Work out the finished part from the listing and answer in its coordinate system (mm). A direction names the side the tool comes from. Round coordinates to 2 decimals unless told otherwise and drop trailing zeros. Write each loop counter-clockwise with the first axis right and the second up, starting at its lowest first coordinate (ties: lowest second). Pieces come first, ordered by that corner, then holes. Notation, with made-up numbers: M 83,-5.75 L 105,-5.75 A23 ccw 105,10.25 Z; hole C 29,7 d9. An arc over 180 degrees is marked long. One line per item, written item: value. Start each with the question number.
Q1. Consider probe 1 along Y at (x, z) = (-234.5, -166); probe 2 along Y at (x, z) = (-195, -372). Determine where each line is inside the solid, lowest interval first.
Q2. Find section C-C (z = -253). Write down the section's boundary in (x, y), and give its area (3 significant figures).
Q3. Given pin 1 Ø6 at (x, y) = (-205.5, 136) entering from -Z; pin 2 Ø16 at (x, z) = (-109.5, -424) entering from -Y; pin 3 Ø4 at (y, z) = (30, -283) entering from +X; pin 4 Ø6 at (x, z) = (-209, -417) entering from +Y, each flat-ended and moving along its own axis, determine where each tip first touches the part or whether it passes through.
Q4. Find section A-A (x = -243.5). Write down the section's boundary in (y, z), and give its area (3 significant figures).
Q5. A tool of negligible diameter and unlimited length cuts with its end or side. For faces 1 (the flat face through (-173, 140, -412)), 2 (the flat face through (-173, 57, -412)), 3 (the flat face through (-350, 59, -309)), from which of +Z, -Z, +X, -X, +Y, -Y can it reach the whole face along a straight path? Write none if from no direction.
Q6. Find section B-B (y = 33.5). Write down the section's boundary in (x, z).
from build123d import *

# Parameters (mm, degrees)
BOSS_EXTRUDE1_DEPTH = 350
SKETCH3_W           = 350
SKETCH3_H           = 15
BOSS_EXTRUDE2_DEPTH = 20


with BuildPart() as part:
    # Sketch1 → Boss-Extrude1 (new body)
    with BuildSketch(Plane(origin=(0, 0, 0), x_dir=(0, 0, -1), z_dir=(1, 0, 0))):
        Polygon((0, 0), (412, 0), (412, 149.955736518), align=None)
    extrude(amount=-BOSS_EXTRUDE1_DEPTH)

    # Sketch3 → Boss-Extrude2 (add)
    with BuildSketch(Plane(origin=(0, 0, -412), x_dir=(-1, 0, 0), z_dir=(0, 0, -1))):
        with Locations((175, 122.455736518)):
            Rectangle(SKETCH3_W, SKETCH3_H)
    extrude(amount=BOSS_EXTRUDE2_DEPTH)


solid = part.part
The answers:
1. probe 1: 0 to 60.42
1. probe 2: 0 to 135.4
2. outline: M -350,0 L 0,0 L 0,92.08 L -350,92.08 Z
2. area: 32,200 mm2
3. pin 1: z = -412
3. pin 2: y = 114.96
3. pin 3: x = 0
3. pin 4: y = 129.96
4. outline: M 0,-412 L 114.96,-412 L 114.96,-432 L 129.96,-432 L 129.96,-412 L 149.96,-412 L 0,0 Z
4. area: 31,200 mm2
5. face 1: -Z, +X, -X, +Y
5. face 2: -Z, +X, -X, -Y
5. face 3: +Z, -Z, -X, +Y, -Y
6. outline: M -350,-412 L 0,-412 L 0,-92.04 L -350,-92.04 Z
